Work out the finished part from the listing and answer in its coordinate system (mm). A direction names the side the tool comes from. Coordinates: 2 decimals unless noted, no trailing zeros. Write each loop counter-clockwise with the first axis right and the second up, starting at its lowest first coordinate (ties: lowest second). Pieces come first, ordered by that corner, then holes. Notation, with made-up numbers: (-10.5, 52) - (11.5, 52) arc R16 ccw to (11.5, 64) - close; hole circle Ø1 at (-27, 57). An arc over 180 degrees is marked (long way). Use a Markdown table: item, result. Add a question column.
(1) Given pin 1 Ø1.5 at (y, z) = (1, -39) entering from +X; pin 2 Ø12 at (x, y) = (-21, 57.5) entering from -Z; pin 3 Ø4.5 at (x, z) = (18.25, 37.2) entering from -Y; pin 4 Ø3 at (x, z) = (23.57, 23.57) entering from +Y, each flat-ended and moving along its own axis, determine where each tip first touches the part or whether it passes through.
(2) For a pull along Y with two mould halves and no side action, classify faces 1 (the face through (-33.2, 41, -23)), 2 (the face through (0, 71.5, 32)), 3 (the face through (-21, 3, -37)) as released by +Y, released by -Y, zero draft, split by the parting line, or undercut.
(3) The part is cut by section D-D, the plane z = -23.57. Give the vertices of the cut face in (x, y).
(4) A tool of negligible diameter and unlimited length cuts with its end or side. For faces 4 (the face through (-21.246, 1, 37)), 5 (the face through (20, 41, -32)), 6 (the face through (-7, 78, -30)), from which of +Z, -Z, +X, -X, +Y, -Y can it reach the whole face along a straight path? Write none if from no direction.
(5) The part is cut by section B-B, the plane y = 46. Give the vertices of the cut face in (x, z).
(6) The part is cut by section A-A, the plane z = 37.2. Give the vertices of the cut face in (x, y), then the cut area to 3 significant figures.
(7) The part is cut by section C-C, the plane x = 0. Give the vertices of the cut face in (y, z), then the cut area to 3 significant figures.
(8) Find the intervals of material crossed by line 1 (X direction, y = 1, z = 37); line 2 (Z direction, x = -21, y = 69); line 3 (Z direction, x = 23, y = 81), in increasing order. Write a range as from..to.
Autodesk Inventor part; units mm, degrees
ref_plane "YZ Plane" through (0, 0, 0) normal (1, 0, 0) x (0, 1, 0)
ref_plane "XZ Plane" through (0, 0, 0) normal (0, 1, 0) x (-1, 0, 0)
ref_plane "XY Plane" through (0, 0, 0) normal (0, 0, 1) x (1, 0, 0)
sketch "Sketch1" plane through (0, 0, 0) normal (0, 1, 0) x (-1, 0, 0)
  line L0 (28.2, -28.2) -> (-28.2, -28.2)
  line L1 (-28.2, -28.2) -> (-28.2, 28.2)
  line L2 (-28.2, 28.2) -> (28.2, 28.2)
  line L3 (28.2, 28.2) -> (28.2, -28.2)
  line L4 (28.2, -28.2) -> (-28.2, 28.2) construction
  line L5 (-28.2, -28.2) -> (28.2, 28.2) construction
  line L6 (33.2, -33.2) -> (-33.2, -33.2)
  line L7 (-33.2, -33.2) -> (-33.2, 33.2)
  line L8 (-33.2, 33.2) -> (33.2, 33.2)
  line L9 (33.2, 33.2) -> (33.2, -33.2)
  line L10 (33.2, -33.2) -> (-33.2, 33.2) construction
  line L11 (-33.2, -33.2) -> (33.2, 33.2) construction
  circle A0 centre (0, 0) radius 20
  line L12 (-21.2465, -33.2) -> (-15.2465, -33.2)
  line L13 (-15.2465, -33.2) -> (-15.2465, -41.2)
  line L14 (-15.2465, -41.2) -> (-21.2465, -41.2)
  line L15 (-21.2465, -41.2) -> (-21.2465, -33.2)
  circle A1 centre (-18.2465, -37.2) radius 2.5
  line L16 (-33.2, 0) -> (33.2, 0) construction
  line L17 (0, -33.2) -> (0, 33.2) construction
  line L18 (-21.2465, 33.2) -> (-15.2465, 33.2)
  line L19 (-15.2465, 33.2) -> (-15.2465, 41.2)
  line L20 (-15.2465, 41.2) -> (-21.2465, 41.2)
  line L21 (-21.2465, 41.2) -> (-21.2465, 33.2)
  circle A2 centre (-18.2465, 37.2) radius 2.5
  line L22 (21.2465, -33.2) -> (15.2465, -33.2)
  line L23 (15.2465, -33.2) -> (15.2465, -41.2)
  line L24 (15.2465, -41.2) -> (21.2465, -41.2)
  line L25 (21.2465, -41.2) -> (21.2465, -33.2)
  circle A3 centre (18.2465, -37.2) radius 2.5
  circle A4 centre (18.2465, 37.2) radius 2.5
  line L26 (15.2465, 33.2) -> (15.2465, 41.2)
  line L27 (15.2465, 41.2) -> (21.2465, 41.2)
  line L28 (21.2465, 41.2) -> (21.2465, 33.2)
  line L29 (21.2465, 33.2) -> (15.2465, 33.2)
  dimension "d0" = 56.4
  dimension "d1" = 5
  dimension "d2" = 5
  dimension "d3" = 40
  dimension "d20" = 6
  dimension "d21" = 5
  dimension "d22" = 3
  dimension "d23" = 4
  dimension "d24" = 8
extrude "Extrusion1" add sketch "Sketch1" along normal blind 3 contours L0 L1 L2 L3 | L6 L7 L8 L9 | L25 L24 L23 L6 | L8 L26 L27 L28 | L13 L14 L15 L6 | L8 L21 L20 L19
sketch "Sketch2" plane through (0, 3, 0) normal (0, 1, 0) x (1, 0, 0)
  line L0 (-33.2, -33.2) -> (-21.2465, -33.2)
  line L1 (33.2, -33.2) -> (33.2, 33.2)
  line L2 (33.2, 33.2) -> (21.2465, 33.2)
  line L3 (-33.2, 33.2) -> (-33.2, -33.2)
  circle A0 centre (0, 0) radius 20
  line L4 (-31, 31) -> (31, 31)
  line L5 (31, 31) -> (31, -31)
  line L6 (31, -31) -> (-31, -31)
  line L7 (-31, -31) -> (-31, 31)
  line L8 (-31, 31) -> (31, -31) construction
  line L9 (31, 31) -> (-31, -31) construction
  line L10 (-21.2465, -33.2) -> (-21.2465, -41.2)
  line L11 (-21.2465, -41.2) -> (-15.2465, -41.2)
  line L12 (-15.2465, -41.2) -> (-15.2465, -33.2)
  line L13 (-15.2465, -33.2) -> (15.2465, -33.2)
  line L14 (15.2465, -33.2) -> (15.2465, -41.2)
  line L15 (15.2465, -41.2) -> (21.2465, -41.2)
  line L16 (21.2465, -41.2) -> (21.2465, -33.2)
  line L17 (21.2465, -33.2) -> (33.2, -33.2)
  line L18 (21.2465, 33.2) -> (21.2465, 41.2)
  line L19 (21.2465, 41.2) -> (15.2465, 41.2)
  line L20 (15.2465, 41.2) -> (15.2465, 33.2)
  line L21 (15.2465, 33.2) -> (-15.2465, 33.2)
  line L22 (-15.2465, 33.2) -> (-15.2465, 41.2)
  line L23 (-15.2465, 41.2) -> (-21.2465, 41.2)
  line L24 (-21.2465, 41.2) -> (-21.2465, 33.2)
  line L25 (-21.2465, 33.2) -> (-33.2, 33.2)
  line L26 (33.2, 33.2) -> (21.2465, 33.2)
  line L27 (15.2465, 41.2) -> (15.2465, 33.2)
  line L28 (33.2, -33.2) -> (33.2, 33.2)
  line L29 (33.2, 33.2) -> (-33.2, 33.2)
  line L30 (21.2465, -33.2) -> (33.2, -33.2)
  line L31 (33.2, -33.2) -> (-33.2, -33.2)
  dimension "d6" = 62
  dimension "d7" = 62
extrude "Extrusion2" add sketch "Sketch2" along normal blind 75 contours L3 L25 L29 L21 L2 L1 L17 L31 L13 L0
sketch "Sketch3" plane through (0, 78, 0) normal (0, 1, 0) x (1, 0, 0)
  line L0 (33.2, -33.2) -> (33.2, 33.2)
  line L1 (33.2, 33.2) -> (-33.2, 33.2)
  line L2 (-33.2, 33.2) -> (-33.2, -33.2)
  line L3 (-33.2, -33.2) -> (33.2, -33.2)
  line L4 (-31, 31) -> (31, 31)
  line L5 (31, 31) -> (31, -31)
  line L6 (31, -31) -> (-31, -31)
  line L7 (-31, -31) -> (-31, 31)
  circle A0 centre (0, 0) radius 28.2247 construction
  circle A1 centre (0, 0) radius 30.2247
  point P0 (-30, 3.4699)
  point P1 (-3.4699, 30)
  point P2 (3.4699, 30)
  point P3 (30, 3.4699)
  point P4 (30, -3.4699)
  point P5 (3.4699, -30)
  point P6 (-3.4699, -30)
  point P7 (-30, -3.4699)
  dimension "d11" = 2
extrude "Extrusion3" add sketch "Sketch3" along normal blind 5 contours L3 L2 L1 L0 | L4 L5 L6 L7
sketch "Sketch4" plane through (0, 83, 0) normal (0, 1, 0) x (1, 0, 0)
  line L0 (33.2, 33.2) -> (-33.2, 33.2)
  line L1 (-33.2, 33.2) -> (-33.2, -33.2)
  line L2 (-33.2, -33.2) -> (33.2, -33.2)
  line L3 (33.2, -33.2) -> (33.2, 33.2)
  line L4 (33.2, -33.2) -> (33.2, 33.2) construction
  line L5 (33.2, 0) -> (-33.2, 0) construction
  line L6 (0, 33.2) -> (0, -33.2) construction
  circle A0 centre (23.57, 23.57) radius 2.3
  circle A1 centre (23.57, -23.57) radius 2.3
  circle A2 centre (-23.57, 23.57) radius 2.3
  circle A3 centre (-23.57, -23.57) radius 2.3
  point P0 (0, 0)
  dimension "d14" = 47.14
  dimension "d15" = 4.6
  dimension "d18" = 47.14
extrude "Extrusion4" cut sketch "Sketch4" against normal blind 10 contours A0 | A1 | A2 | A3
sketch "Sketch5" plane through (33.2, 0, 33.2) normal (1, 0, 0) x (0, 0, -1)
  line L0 (-8, 0) -> (0, 0)
  line L1 (-8, 0) -> (0, 0)
  line L2 (0, 0) -> (0, 3)
  line L3 (-8, 3) -> (0, 3)
  line L4 (-8, 0) -> (-8, 3)
  line L5 (0, 0) -> (66.4, 0)
  line L6 (66.4, 0) -> (66.4, 83)
  line L7 (0, 83) -> (66.4, 83)
  line L8 (0, 0) -> (0, 83)
  line L9 (66.4, 3) -> (74.4, 3)
  line L10 (66.4, 0) -> (74.4, 0)
  line L11 (66.4, 0) -> (74.4, 0)
  line L12 (74.4, 0) -> (74.4, 3)
  line L13 (66.4, 3) -> (74.4, 3)
  line L14 (66.4, 0) -> (66.4, 3)
  line L15 (74.4, 3) -> (66.4, 3) construction
  line L16 (0, 3) -> (66.4, 3) construction
  line L17 (33.2, 0) -> (33.2, 83) construction
  line L18 (0, 0) -> (0, 83) construction
  line L19 (0, 41.5) -> (66.4, 41.5) construction
  line L20 (66.4, 0) -> (66.4, 83) construction
  line L21 (13.2, 71.5) -> (53.2, 71.5)
  line L22 (53.2, 71.5) -> (53.2, 11.5)
  line L23 (53.2, 11.5) -> (13.2, 11.5)
  line L24 (13.2, 11.5) -> (13.2, 71.5)
  line L25 (13.2, 71.5) -> (53.2, 11.5) construction
  line L26 (53.2, 71.5) -> (13.2, 11.5) construction
  point P0 (33.2, 41.5)
  dimension "d27" = 40
  dimension "d28" = 60
extrude "Extrusion5" cut sketch "Sketch5" against normal through all contours L21 L22 L23 L24
sketch "Sketch6" plane through (15.2465, 0, -33.2) normal (0, 0, -1) x (-1, 0, 0)
  line L0 (-17.9535, 0) -> (-6, 0)
  line L1 (-6, 0) -> (-6, 3)
  line L2 (0, 3) -> (-6, 3)
  line L3 (0, 0) -> (0, 3)
  line L4 (0, 0) -> (30.493, 0)
  line L5 (30.493, 0) -> (30.493, 3)
  line L6 (36.493, 3) -> (30.493, 3)
  line L7 (36.493, 0) -> (36.493, 3)
  line L8 (36.493, 0) -> (48.4465, 0)
  line L9 (48.4465, 0) -> (48.4465, 83)
  line L10 (-17.9535, 83) -> (48.4465, 83)
  line L11 (-17.9535, 0) -> (-17.9535, 83)
  line L12 (-17.9535, 11.5) -> (-17.9535, 71.5) construction
  line L13 (-17.9535, 41.5) -> (48.4465, 41.5) construction
  line L14 (48.4465, 0) -> (48.4465, 83) construction
  line L15 (48.4465, 83) -> (-17.9535, 83) construction
  line L16 (15.2465, 83) -> (15.2465, 0) construction
  line L17 (-4.7535, 71.5) -> (35.2465, 71.5)
  line L18 (35.2465, 71.5) -> (35.2465, 11.5)
  line L19 (35.2465, 11.5) -> (-4.7535, 11.5)
  line L20 (-4.7535, 11.5) -> (-4.7535, 71.5)
  line L21 (-4.7535, 71.5) -> (35.2465, 11.5) construction
  line L22 (35.2465, 71.5) -> (-4.7535, 11.5) construction
  point P0 (15.2465, 41.5)
  dimension "d29" = 40
  dimension "d30" = 60
extrude "Extrusion6" cut sketch "Sketch6" against normal up to surface (66.4 mm away) contours L17 L18 L19 L20
properties part number "Motor case"
Model answer:
| question | item | result |
|---|---|---|
| 1 | pin 1 | x = 21.25 |
| 1 | pin 2 | z = -33.2 |
| 1 | pin 3 | through |
| 1 | pin 4 | y = 3 |
| 2 | face 1 | zero draft |
| 2 | face 2 | undercut |
| 2 | face 3 | released by +Y |
| 3 | outline | (-33.2, 0) - (33.2, 0) - (33.2, 83) - (25.87, 83) - (25.87, 78) - (31, 78) - (31, 3) - (-31, 3) - (-31, 78) - (-25.87, 78) - (-25.87, 83) - (-33.2, 83) - close; (-21.27, 78) - (-18.92, 78) - (-18.92, 83) - (-21.27, 83) - close; (18.92, 78) - (21.27, 78) - (21.27, 83) - (18.92, 83) - close |
| 4 | face 4 | +Z, -X, +Y, -Y |
| 4 | face 5 | +Z, -Z |
| 4 | face 6 | none |
| 5 | outline | (-33.2, -33.2) - (-20, -33.2) - (-20, -31) - (-31, -31) - (-31, -20) - (-33.2, -20) - close; (-33.2, 20) - (-31, 20) - (-31, 31) - (-20, 31) - (-20, 33.2) - (-33.2, 33.2) - close; (20, -33.2) - (33.2, -33.2) - (33.2, -20) - (31, -20) - (31, -31) - (20, -31) - close; (20, 31) - (31, 31) - (31, 20) - (33.2, 20) - (33.2, 33.2) - (20, 33.2) - close |
| 6 | outline | (-21.25, 0) - (-20.75, 0) - (-20.75, 3) - (-21.25, 3) - close; (-15.75, 0) - (-15.25, 0) - (-15.25, 3) - (-15.75, 3) - close; (15.25, 0) - (15.75, 0) - (15.75, 3) - (15.25, 3) - close; (20.75, 0) - (21.25, 0) - (21.25, 3) - (20.75, 3) - close |
| 6 | area | 6.00 mm^2 |
| 7 | outline | (0, -33.2) - (11.5, -33.2) - (11.5, -31) - (3, -31) - (3, -20) - (0, -20) - close; (0, 20) - (3, 20) - (3, 31) - (11.5, 31) - (11.5, 33.2) - (0, 33.2) - close; (71.5, -33.2) - (83, -33.2) - (83, -30.22) - (78, -30.22) - (78, -31) - (71.5, -31) - close; (71.5, 31) - (78, 31) - (78, 30.22) - (83, 30.22) - (83, 33.2) - (71.5, 33.2) - close |
| 7 | area | 175 mm^2 |
| 8 | line 1 | -21.25..-20.74, -15.75..-15.25, 15.25..15.75, 20.74..21.25 |
| 8 | line 2 | -33.2..-31, 31..33.2 |
| 8 | line 3 | -33.2..-25.8, -21.34..-19.61, 19.61..21.34, 25.8..33.2 |
